Design review of the part built by this model. Coordinates are the model's own, in mm. A direction names the side the tool comes from. Coordinates: 2 decimals unless noted, no trailing zeros. Write each loop counter-clockwise with the first axis right and the second up, starting at its lowest first coordinate (ties: lowest second). Pieces come first, ordered by that corner, then holes. Notation, with made-up numbers: M 70,54.5 L 104,54.5 A23 ccw 104,83.5 Z; hole C -7.5,73.25 d5. An arc over 180 degrees is marked long. Write item = value, one per line.
```python
from build123d import *

# Parameters (mm, degrees)
CROQUIS1_R                 = 30
SALIENTE_EXTRUIR1_DEPTH    = 20
CORTAR_EXTRUIR1_DEPTH      = 47.904157598
CORTAR_EXTRUIR1_DEPTH_BACK = 47.904157598
CROQUIS2_W                 = 30
CROQUIS2_H                 = 17
CORTAR_EXTRUIR2_DEPTH      = 47.904157598
CORTAR_EXTRUIR2_DEPTH_BACK = 47.904157598
CROQUIS3_W                 = 30
CROQUIS3_H                 = 17


with BuildPart() as part:
    # Croquis1 → Saliente-Extruir1 (new body)
    with BuildSketch(Plane(origin=(0, 0, 0), x_dir=(1, 0, 0), z_dir=(0, 1, 0))):
        with Locations(Location((0, 0, 0), (0, 0, 270))):
            Circle(CROQUIS1_R)
    extrude(amount=SALIENTE_EXTRUIR1_DEPTH)

    # Croquis2 → Cortar-Extruir1 (cut, two sides: drawn at the far end of the back side and taken through both)
    with BuildSketch(Plane.XY.offset(-CORTAR_EXTRUIR1_DEPTH_BACK)):
        with Locations((0, 8.5)):
            Rectangle(CROQUIS2_W, CROQUIS2_H)
    extrude(amount=CORTAR_EXTRUIR1_DEPTH + CORTAR_EXTRUIR1_DEPTH_BACK, mode=Mode.SUBTRACT)

    # Croquis3 → Cortar-Extruir2 (cut, two sides: drawn at the far end of the back side and taken through both)
    with BuildSketch(Plane(origin=(0, 0, 0), x_dir=(0, 0, -1), z_dir=(1, 0, 0)).offset(-CORTAR_EXTRUIR2_DEPTH_BACK)):
        with Locations((0, 8.5)):
            Rectangle(CROQUIS3_W, CROQUIS3_H)
    extrude(amount=CORTAR_EXTRUIR2_DEPTH + CORTAR_EXTRUIR2_DEPTH_BACK, mode=Mode.SUBTRACT)


solid = part.part
```
Q1. Consider section C-C, the plane x = -16.5. State the section outline as (y, z) points, and give its area (3 significant figures).
Check result:
outline = M 0,-25.05 L 20,-25.05 L 20,25.05 L 0,25.05 L 0,15 L 17,15 L 17,-15 L 0,-15 Z
area = 492 mm²
Q2. Consider section B-B, the plane z = -23.5. State the section outline as (x, y) points.
Check result:
outline = M -18.65,0 L -15,0 L -15,17 L 15,17 L 15,0 L 18.65,0 L 18.65,20 L -18.65,20 Z
Q3. For P1, Ø5.5, axis at y = 11.5, z = 18.5, coming from the -X side; P2, Ø5.5, axis at x = -21.5, y = 10, coming from the -Z side; P3, Ø3.5, axis at y = 11, z = 22.5, coming from the +X side, all flat-tipped, find the tip position at first contact; note any pin that passes through.
Check result:
P1 = -25.53
P2 = -23.42
P3 = 21.67
Q4. Machinability: for faces 1 (the flat face through (-15, 8, 20)), 2 (the flat face through (19, 0, -19)), 3 (the flat face through (-21, 8, 15)), which of the approach directions +Z, -Z, +X, -X, +Y, -Y give a long, thin tool a straight path to every point of the face, cutting with its end or side? Answer none if there is none.
Check result:
face_1 = +Z, -Z, -Y
face_2 = +Z, -Z, +X, -X, -Y
face_3 = +X, -X, -Y
Q5. The part is to be moulded in two halves that separate along X. For faces 4 (the flat face through (15, 8, 20)), 5 (the cylindrical face through (20.275, 12.082, -22.111)), 6 (the flat face through (20, 8, 15)), say which applies: +X half, -X half, draft (parallel to the pull), parting line (faces both ways), or undercut.
Check result:
face_4 = undercut
face_5 = parting line
face_6 = draft
Q6. Wall thickness on line 1 (Y direction, x = 12, z = -15); line 2 (X direction, y = 5.75, z = -23.5); line 3 (Z direction, x = 22, y = 4.25): over which ranges is each line inside the solid? List them lowest first.
Check result:
line_1 = 17 to 20
line_2 = -18.65 to -15, 15 to 18.65
line_3 = -20.4 to -15, 15 to 20.4
Q7. Consider section D-D, the plane z = 0. State the section outline as (x, y) points, and give its area (3 significant figures).
Check result:
outline = M -30,17 L 30,17 L 30,20 L -30,20 Z
area = 180 mm²
Q8. Consider section A-A, the plane y = 2.5. State the section outline as (x, z) points.
Check result:
outline = M -25.98,-15 A30 ccw -15,-25.98 L -15,-15 Z; M -25.98,15 L -15,15 L -15,25.98 A30 ccw Z; M 15,-25.98 A30 ccw 25.98,-15 L 15,-15 Z; M 15,15 L 25.98,15 A30 ccw 15,25.98 Z
